```python
from build123d import *

# Parameters (mm, degrees)
SKETCH1_W      = 28
SKETCH1_H      = 9
EXTRUDE1_DEPTH = 19
SKETCH2_R      = 1.6
EXTRUDE2_DEPTH = 26.621437653
SKETCH3_W      = 19.5
SKETCH3_H      = 15
EXTRUDE3_DEPTH = 27.643580689
SKETCH6_R      = 1.6
EXTRUDE4_DEPTH = 3
EXTRUDE5_START = 3
SKETCH7_R      = 1.6
EXTRUDE5_DEPTH = 3
SKETCH8_W      = 6.6
SKETCH8_H      = 6.4
EXTRUDE6_DEPTH = 1
SKETCH9_R      = 1.55
EXTRUDE7_DEPTH = 27.322621297
FILLET1_R      = 1


with BuildPart() as part:
    # Sketch1 → Extrude1 (new body)
    with BuildSketch(Plane(origin=(0, 0, 0), x_dir=(1, 0, 0), z_dir=(0, 1, 0))):
        with Locations((2.367052023, 0.751445087)):
            Rectangle(SKETCH1_W, SKETCH1_H)
    extrude(amount=EXTRUDE1_DEPTH)

    # Sketch2 → Extrude2 (cut, through all)
    with BuildSketch(Plane(origin=(0, 19, 0), x_dir=(1, 0, 0), z_dir=(0, 1, 0))):
        with Locations(Location((-0.632947977, 0.751445087, 0), (0, 0, 270))):
            Circle(SKETCH2_R)
    extrude(amount=-EXTRUDE2_DEPTH, mode=Mode.SUBTRACT)

    # Sketch3 → Extrude3 (cut, through all)
    with BuildSketch(Plane.XY.offset(3.748554913)):
        with Locations((-1.882947977, 9.5)):
            Rectangle(SKETCH3_W, SKETCH3_H)
    extrude(amount=-EXTRUDE3_DEPTH, mode=Mode.SUBTRACT)

    # Sketch6 → Extrude4 (add)
    with BuildSketch(Plane(origin=(0, 2, 0), x_dir=(1, 0, 0), z_dir=(0, 1, 0))):
        with Locations(Location((-6.132947977, 0.751445087, 0), (0, 0, 90))):
            Circle(SKETCH6_R)
    extrude(amount=EXTRUDE4_DEPTH)

    # Sketch7 → Extrude5 (add)
    with BuildSketch(Plane.XZ.offset(-17).offset(EXTRUDE5_START)):
        with Locations(Location((-6.132947977, -0.751445087, 0), (0, 0, 270))):
            Circle(SKETCH7_R)
    extrude(amount=-EXTRUDE5_DEPTH)

    # Sketch8 → Extrude6 (cut)
    with BuildSketch(Plane(origin=(0, 0, -5.251445087), x_dir=(-1, 0, 0), z_dir=(0, 0, -1))):
        with Locations((-13.067052023, 9.5)):
            Rectangle(SKETCH8_W, SKETCH8_H)
    extrude(amount=-EXTRUDE6_DEPTH, mode=Mode.SUBTRACT)

    # Sketch9 → Extrude7 (cut, through all)
    with BuildSketch(Plane(origin=(0, 0, -4.251445087), x_dir=(-1, 0, 0), z_dir=(0, 0, -1))):
        with Locations((-13.373052023, 9.5)):
            Circle(SKETCH9_R)
    extrude(amount=-EXTRUDE7_DEPTH, mode=Mode.SUBTRACT)

    # Fillet1
    fillet1_edges = [part.edges().sort_by_distance(p)[0] for p in [
        (2.367052023, 19, -5.251445087),
        (2.367052023, 0, 3.748554913),
        (2.367052023, 0, -5.251445087),
        (16.367052023, 0, -0.751445087),
        (16.367052023, 3.15, -5.251445087),
        (16.367052023, 9.5, 3.748554913),
        (-11.632947977, 0, -0.751445087),
        (-1.882947977, 2, 3.748554913),
        (-1.882947977, 2, -5.251445087),
        (7.867052023, 2, -0.751445087),
        (7.867052023, 17, -0.751445087),
        (7.867052023, 9.5, -5.251445087),
        (-1.882947977, 17, -5.251445087),
        (-11.632947977, 19, -0.751445087),
        (7.867052023, 9.5, 3.748554913),
        (-1.882947977, 17, 3.748554913),
        (2.367052023, 19, 3.748554913),
        (16.367052023, 19, -0.751445087),
        (16.367052023, 15.85, -5.251445087),
        (-11.632947977, 1, -5.251445087),
        (-11.632947977, 1, 3.748554913),
        (-11.632947977, 18, -5.251445087),
        (-11.632947977, 18, 3.748554913),
    ]]
    fillet(fillet1_edges, radius=FILLET1_R - 0.0001)  # a hair under: the kernel refuses the full size


solid = part.part
```
Geometry check sheet. Reference: the model listing, model coordinates, mm. A direction names the side the tool comes from. Round coordinates to 2 decimals unless told otherwise and drop trailing zeros. Order: outer loops, then holes, each group sorted by start corner. A loop starts at its lowest first (then second) coordinate and runs counter-clockwise, first axis right, second up. Notation, with made-up numbers: M -9,50 L 38,50 A27 cw 38,85 Z; hole C 40.5,34 d6. An arc over 180 degrees is marked long. Write item = value, one per line.
Q1. Depth check by flat-ended pin: pin 1 Ø2 at (y, z) = (14.5, 2.5) entering from -X; pin 2 Ø2.5 at (x, y) = (13.37, 9.5) entering from -Z; pin 3 Ø0.8 at (x, z) = (12.5, -5) entering from -Y; pin 4 Ø5 at (x, y) = (13, 9) entering from -Z. Enter the tip coordinate at first touch or a pass-through.
Answer block:
pin_1 = 7.87
pin_2 = through
pin_3 = 0.06
pin_4 = -4.25
Q2. Section check D-D (z = -3.5). Enter the section's corners in (x, y).
Answer block:
outline = M -11.63,1 A1 ccw -10.63,0 L 15.37,0 A1 ccw 16.37,1 L 16.37,18 A1 ccw 15.37,19 L -10.63,19 A1 ccw -11.63,18 L -11.63,17 L 6.87,17 A1 cw 7.87,16 L 7.87,3 A1 cw 6.87,2 L -11.63,2 Z; hole C 13.37,9.5 d3.1
Q3. Set-up check for faces 1 (the flat face through (-6, 5, -1)), 2 (the cylindrical face through (-4.547, 15.479, -0.543)), 3 (the cylindrical face through (-2.25, 1.71, 3.45)), 4 (the flat face through (11.6, 9.5, -4.251)): record each of +Z, -Z, +X, -X, +Y, -Y from which the full face is reachable in a straight line by a thin tool's end or side.
Answer block:
face_1 = +Z, -Z, -X
face_2 = none
face_3 = +Z, -X
face_4 = -Z, +X
Q4. Section check A-A (y = 9.5). Enter the section's corners in (x, z).
Answer block:
outline = M 7.87,-4.25 A1 ccw 8.87,-5.25 L 9.77,-5.25 L 9.77,-4.25 L 11.82,-4.25 L 11.82,3.75 L 8.87,3.75 A1 ccw 7.87,2.75 Z; M 14.92,-4.25 L 16.37,-4.25 L 16.37,2.75 A1 ccw 15.37,3.75 L 14.92,3.75 Z
Q5. Release check for a two-part mould opening along X. For faces 5 (the flat face through (13, 12.7, -5)), 6 (the cylindrical face through (-1.61, 18.01, -2.02)), 7 (the cylindrical face through (16.07, 9.62, 3.46)) record: released by +X, released by -X, zero draft, split by the parting line, or undercut.
Answer block:
face_5 = zero draft
face_6 = undercut
face_7 = released by +X
Q6. Scan lines: line 1 (Y direction, x = 0, z = 1.25); line 2 (X direction, y = 9, z = -2.5); line 3 (Z direction, x = 12, y = 11). Record each from-to range of solid material in increasing order.
Answer block:
line_1 = 0 to 2, 17 to 19
line_2 = 7.87 to 11.91, 14.84 to 16.37
line_3 = -4.25 to 3.75
Q7. Section check B-B (z = -0.75). Give the number of separate pieces and of enclosed holes in the cut face, plus the area to 3 significant figures.
Answer block:
separate_pieces = 3
enclosed_holes = 1
area = 238 mm^2
